Job drawing, mm, ordinate dimensions from the low corner. One solid piece. A direction names the side the tool comes from. Give positions to 0.01 mm unless a question says otherwise; leave off trailing zeros. Order: outer loops, then holes, each group sorted by start corner. A loop starts at its lowest first (then second) coordinate and runs counter-clockwise, first axis right, second up.
Item 1: Band-saw the part on D-D on x = 12.5. Give the cut face in (y, z).
Item 2: Band-saw the part on B-B on x = 18.75. Give the cut face in (y, z).
Item 3: Wall check: L1, parallel to X at y = 32.5, z = 1.5; L2, parallel to Y at x = 2.5, z = 1.65; L3, parallel to Y at x = 11.25, z = 1.9 (1 decimal). Give the ranges that are in metal, low to high.
Item 4: Which spindle directions (+Z, -Z, +X, -X, +Y, -Y) get a long thin tool onto all of the face, cutting with end or side? Do the marked faces 4, 5 and 6. Say none if no direction does.
Item 5: Band-saw the part on A-A on y = 32.5. Give the cut face in (x, z).
Item 6: Flat gauge pins, fed straight in: P1, Ø0.9, axis at x = 20.49, y = 32.5, coming from the -Z side; P2, Ø1.5, axis at x = 8.5, z = 2.5, coming from the +Y side. Where does each tip first touch, or does it go through?
Item 7: Band-saw the part on C-C on z = 2.2. Give the cut face in (x, y) (1 decimal), plus the area to 3 significant figures.
Item 8: Two-plate mould, pull along X, no slides. Class the marked faces 1, 2 and 3: released by +X, released by -X, zero draft, split by the parting line, or undercut.
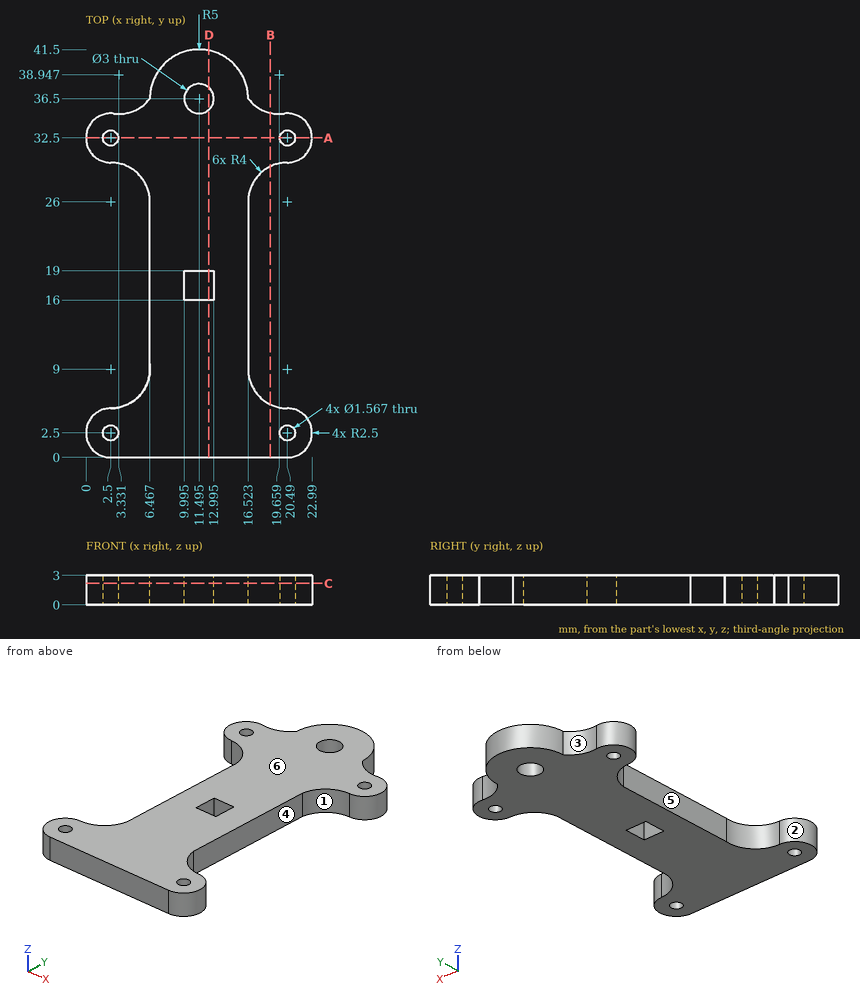
The answers:
1. outline: (0, 0) - (16, 0) - (16, 3) - (0, 3) - close; (19, 0) - (35.39, 0) - (35.39, 3) - (19, 3) - close; (37.61, 0) - (41.4, 0) - (41.4, 3) - (37.61, 3) - close
2. outline: (0, 0) - (5.4, 0) - (5.4, 3) - (0, 3) - close; (29.6, 0) - (35.05, 0) - (35.05, 3) - (29.6, 3) - close
3. L1: x = 0 to 1.72, 3.28 to 19.71, 21.27 to 22.99
3. L2: y = 0 to 1.72, 3.28 to 5, 30 to 31.72, 33.28 to 35
3. L3: y = 0 to 16, 19 to 35, 38 to 41.5
4. face 4: +Z, -Z, +X
4. face 5: +Z, -Z, -X
4. face 6: +Z, +X, -X, +Y, -Y
5. outline: (0, 0) - (1.72, 0) - (1.72, 3) - (0, 3) - close; (3.28, 0) - (19.71, 0) - (19.71, 3) - (3.28, 3) - close; (21.27, 0) - (22.99, 0) - (22.99, 3) - (21.27, 3) - close
6. P1: passes through
6. P2: stops at y = 40.97
7. outline: (2.5, 0) - (20.5, 0) arc R2.5 ccw to (20.5, 5) arc R4 cw to (16.5, 8.5) - (16.5, 26.5) arc R4 cw to (20.5, 30) arc R2.5 ccw (long way) to (20.2, 35) arc R4 cw to (16.5, 36.5) arc R5 ccw to (6.5, 36.5) arc R4 cw to (2.8, 35) arc R2.5 ccw (long way) to (2.5, 30) arc R4 cw to (6.5, 26.5) - (6.5, 9.5) arc R4 cw to (2.5, 5) arc R2.5 ccw to start; hole circle Ø1.6 at (2.5, 2.5); hole circle Ø1.6 at (2.5, 32.5); hole (10, 16) - (13, 16) - (13, 19) - (10, 19) - close; hole circle Ø3 at (11.5, 36.5); hole circle Ø1.6 at (20.5, 2.5); hole circle Ø1.6 at (20.5, 32.5)
7. area: 517 mm2
8. face 1: released by +X
8. face 2: released by -X
8. face 3: undercut
